Here's the drawing with two shaded views (mm, measured from the low corner). I have some questions. A direction names the side the tool comes from. Round coordinates to 2 decimals unless told otherwise and drop trailing zeros. Loops run counter-clockwise (first coordinate to the right, second up) from the corner with the lowest first, then second, coordinate; pieces in that order, holes last. Notation, with made-up numbers: (-1, -37) -> (9, -37) arc R24 ccw to (9, -25) -> close; hole circle Ø9 at (-22, 56). An arc over 180 degrees is marked (long way). Write item = value, one per line.
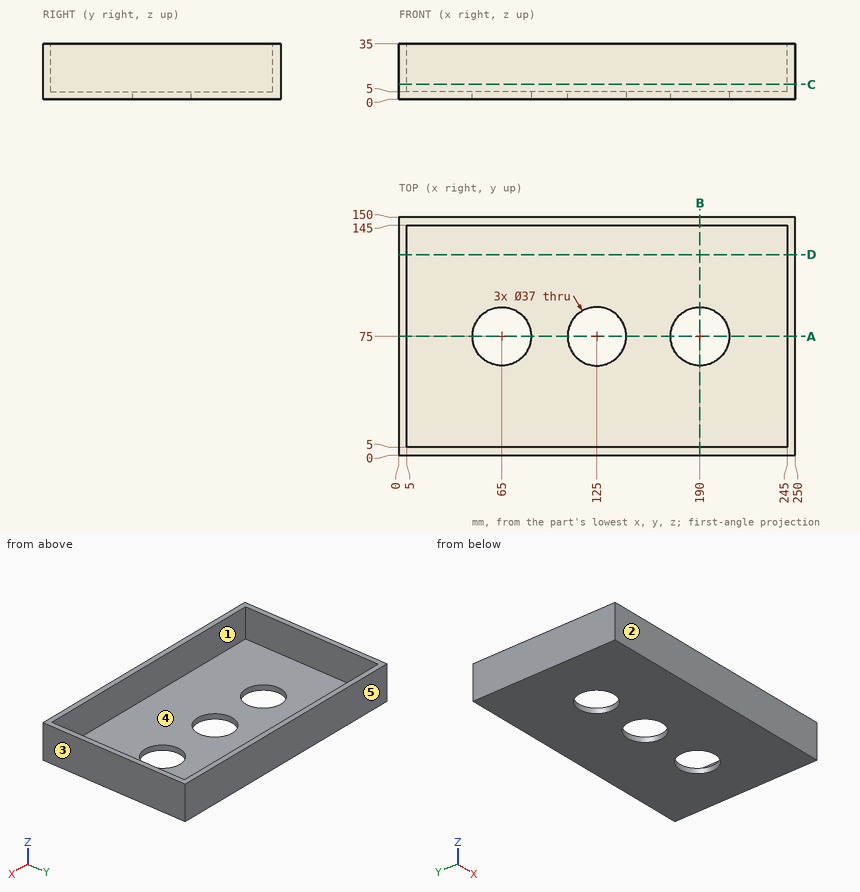
1. Suppose I cut it at B-B, the plane x = 190. List the corners of the cut face in (y, z) for me, and give its area (3 significant figures).
Entries:
outline = (0, 0) -> (56.5, 0) -> (56.5, 5) -> (5, 5) -> (5, 35) -> (0, 35) -> close; (93.5, 0) -> (150, 0) -> (150, 35) -> (145, 35) -> (145, 5) -> (93.5, 5) -> close
area = 865 mm²
2. For the marked faces 1 and 2, which set-ups out of +Z, -Z, +X, -X, +Y, -Y let a thin tool reach every point of the face, with its end or its side?
Entries:
face_1 = +Z
face_2 = +Z, -Z, +X, -X, -Y
3. Suppose I cut it at C-C, the plane z = 9.5. List the corners of the cut face in (x, y) for me, and give its area (3 significant figures).
Entries:
outline = (0, 0) -> (250, 0) -> (250, 150) -> (0, 150) -> close; hole (5, 5) -> (245, 5) -> (245, 145) -> (5, 145) -> close
area = 3,900 mm²
4. I'm going to push a flat-ended pin straight in: pin 1 (1 mm diameter, centred on x = 146.5, z = 28.5, fed in from -Y). Where does the tip first touch, or does it pass through?
Entries:
pin_1 = 0
5. I need wall thicknesses on line 1 (Y direction, x = 179, z = 33); line 2 (Y direction, x = 190, z = 2.2); line 3 (Z direction, x = 92.5, y = 94). Which ranges of each line are inside material? Lowest first, please. Write a range as [from, to].
Entries:
line_1 = [0, 5], [145, 150]
line_2 = [0, 56.5], [93.5, 150]
line_3 = [0, 5]
6. Suppose I cut it at D-D, the plane y = 126.5. List the corners of the cut face in (x, z) for me.
Entries:
outline = (0, 0) -> (250, 0) -> (250, 35) -> (245, 35) -> (245, 5) -> (5, 5) -> (5, 35) -> (0, 35) -> close
7. Suppose I cut it at A-A, the plane y = 75. List the corners of the cut face in (x, z) for me, and give its area (3 significant figures).
Entries:
outline = (0, 0) -> (46.5, 0) -> (46.5, 5) -> (5, 5) -> (5, 35) -> (0, 35) -> close; (83.5, 0) -> (106.5, 0) -> (106.5, 5) -> (83.5, 5) -> close; (143.5, 0) -> (171.5, 0) -> (171.5, 5) -> (143.5, 5) -> close; (208.5, 0) -> (250, 0) -> (250, 35) -> (245, 35) -> (245, 5) -> (208.5, 5) -> close
area = 995 mm²
8. We'd pull the mould along X, two halves only. Please class the marked faces 3, 4 and 5: released by +X, released by -X, zero draft, split by the parting line, or undercut.
Entries:
face_3 = released by +X
face_4 = undercut
face_5 = zero draft
